from build123d import *

# Parameters (mm, degrees)
SKETCH_1_R          = 14
EXTRUDE_1_DEPTH     = 2.5
CHAMFER_4_SIZE      = 0.5
CHAMFER_4_SIZE2     = 1.37373871
SKETCH_3_W          = 19.861324318
SKETCH_3_H          = 0.4
CUT_EXTRUDE_1_DEPTH = 20.956202044
CHAMFER_5_SIZE      = 1
CHAMFER_5_SIZE2     = 0.363970234


with BuildPart() as part:
    # Эскиз1 → Бобышка-Вытянуть1 (new body)
    with BuildSketch(Plane(origin=(0, 0, 0), x_dir=(1, 0, 0), z_dir=(0, 1, 0))):
        with Locations(Location((0, -1e-09, 0), (0, 0, 270))):
            Circle(SKETCH_1_R)
        with BuildLine():
            Line((-6.907932165, 5.768923055), (-1.542067835, 8.866906269))
            ThreePointArc((-1.542067835, 8.866906269), (0, 9), (1.542067835, 8.866906269))
            Line((1.542067835, 8.866906269), (6.907932165, 5.768923055))
            ThreePointArc((6.907932165, 5.768923055), (7.794228634, 4.5), (8.45, 3.097983215))
            Line((8.45, 3.097983215), (8.45, -3.097983215))
            ThreePointArc((8.45, -3.097983215), (7.794228634, -4.5), (6.907932165, -5.768923055))
            Line((6.907932165, -5.768923055), (1.542067835, -8.866906269))
            ThreePointArc((1.542067835, -8.866906269), (0, -9), (-1.542067835, -8.866906269))
            Line((-1.542067835, -8.866906269), (-6.907932165, -5.768923054))
            ThreePointArc((-6.907932165, -5.768923054), (-7.794228634, -4.5), (-8.45, -3.097983215))
            Line((-8.45, -3.097983215), (-8.45, 3.097983215))
            ThreePointArc((-8.45, 3.097983215), (-7.794228634, 4.5), (-6.907932165, 5.768923055))
        make_face(mode=Mode.SUBTRACT)
    extrude(amount=EXTRUDE_1_DEPTH)

    # Фаска4
    chamfer_4_edges = [part.edges().sort_by_distance(p)[0] for p in [
        (-7.794228634, 2.5, -4.5),
        (-8.45, 2.5, 0),
        (-7.794228634, 2.5, 4.5),
        (-4.225, 2.5, 7.317914662),
        (0, 2.5, 9),
        (4.225, 2.5, 7.317914662),
        (7.794228634, 2.5, 4.5),
        (8.45, 2.5, 0),
        (7.794228634, 2.5, -4.5),
        (4.225, 2.5, -7.317914662),
        (0, 2.5, -9),
        (-4.225, 2.5, -7.317914662),
    ]]
    chamfer_4_side = [part.faces().sort_by_distance(p)[0] for p in [
        (0, 2.5, -13.604020202),
    ]]
    chamfer(chamfer_4_edges, length=CHAMFER_4_SIZE, length2=CHAMFER_4_SIZE2, reference=chamfer_4_side[0])

    # Эскиз3 → Вырез-Вытянуть1 (cut, through all)
    with BuildSketch(Plane(origin=(0, 2.5, 0), x_dir=(1, 0, 0), z_dir=(0, 1, 0))):
        with Locations((-7.474129941, 0)):
            Rectangle(SKETCH_3_W, SKETCH_3_H)
    extrude(amount=-CUT_EXTRUDE_1_DEPTH, mode=Mode.SUBTRACT)

    # Фаска5
    chamfer_5_edges = [part.edges().sort_by_distance(p)[0] for p in [
        (9.969954865, 2.5, -9.828529899),
    ]]
    chamfer_5_side = [part.faces().sort_by_distance(p)[0] for p in [
        (9.969954865, 1.25, -9.828529899),
    ]]
    chamfer(chamfer_5_edges, length=CHAMFER_5_SIZE, length2=CHAMFER_5_SIZE2, reference=chamfer_5_side[0])


solid = part.part
The listing builds one solid part. Answer for the finished solid, in the listing's coordinates (mm). A direction names the side the tool comes from. Round coordinates to 2 decimals unless told otherwise and drop trailing zeros. Order: outer loops, then holes, each group sorted by start corner. A loop starts at its lowest first (then second) coordinate and runs counter-clockwise, first axis right, second up. Notation, with made-up numbers: (73.25, 86.5) - (90.25, 86.5) arc R19 ccw to (90.25, 108.5) - close; hole circle Ø10 at (66, 68). An arc over 180 degrees is marked (long way). Write item = value, one per line. Start each with the question number.
1) Given pin 1 (0.9 mm diameter, centred on y = 0.5, z = 2.5, fed in from +X); pin 2 (1.3 mm diameter, centred on x = -11.5, y = 1.5, fed in from +Z); pin 3 (1.2 mm diameter, centred on x = -10.5, y = 1.5, fed in from -Z), each flat-ended and moving along its own axis, determine where each tip first touches the part or whether it passes through.
2) Section A-A, the plane y = 0.65 is taken. Write down the section's boundary in (x, z).
3) Straight lines are drawn through the part: L1, parallel to Z at x = 0.25, y = 0.3; L2, parallel to Z at x = 2.75, y = 2.1; L3, parallel to X at y = 0.6, z = -2.25. For each, find the intervals that lie inside material, in ascending order.
4) For a pull along Z with two mould halves and no side action, classify faces 1 (the flat face through (6.4, 0, -6.4)), 2 (the cylindrical face through (-7.805, 0.555, -4.481)) as released by +Z, released by -Z, zero draft, split by the parting line, or undercut.
5) For faces 3 (the flat face through (4.26, 0.56, 7.3)), 4 (the flat face through (9.3, 2.5, -0.2)), 5 (the flat face through (-4.31, 1.8, 7.55)), determine the directions among +Z, -Z, +X, -X, +Y, -Y from which every point of the face is accessible in a straight line to the end or side of a thin tool.
Results list:
q1.pin_1 = 13.85
q1.pin_2 = 8.85
q1.pin_3 = -9.9
q2.outline = (-14, -0.2) arc R14 ccw (long way) to (-14, 0.2) - (-8.45, 0.2) - (-8.45, 3.1) arc R9 cw to (-6.91, 5.77) - (-1.54, 8.87) arc R9 cw to (1.54, 8.87) - (6.91, 5.77) arc R9 cw to (8.45, 3.1) - (8.45, -3.1) arc R9 cw to (6.91, -5.77) - (1.54, -8.87) arc R9 cw to (-1.54, -8.87) - (-6.91, -5.77) arc R9 cw to (-8.45, -3.1) - (-8.45, -0.2) - close
q3.L1 = -14 to -9, 9 to 14
q3.L2 = -13.5 to -8.58, 8.58 to 13.5
q3.L3 = -13.82 to -8.45, 8.45 to 13.82
q4.face_1 = zero draft
q4.face_2 = undercut
q5.face_3 = +Y, -Y
q5.face_4 = +Z, -Z, +X, -X, +Y
q5.face_5 = +Y
